Check sheet for the modelled part. Datum: model origin and axes. Units: mm. Face numbers are marked on the shaded views. A direction names the side the tool comes from. Give positions to 0.01 mm unless a question says otherwise; leave off trailing zeros. Loops run counter-clockwise (first coordinate to the right, second up) from the corner with the lowest first, then second, coordinate; pieces in that order, holes last. Notation, with made-up numbers: M -0.75,10 L 35.25,10 A25 cw 35.25,47 Z; hole C -23,6.5 d4. An arc over 180 degrees is marked long. Use one line per item in the form item = value.
Autodesk Inventor part; units mm, degrees
ref_plane "YZ Plane" through (0, 0, 0) normal (1, 0, 0) x (0, 1, 0)
ref_plane "XZ Plane" through (0, 0, 0) normal (0, 1, 0) x (-1, 0, 0)
ref_plane "XY Plane" through (0, 0, 0) normal (0, 0, 1) x (1, 0, 0)
sketch "Sketch1" plane through (0, 0, 0) normal (0, 1, 0) x (-1, 0, 0)
  line L0 (-8.75, 22.75) -> (8.75, 22.75)
  line L1 (8.75, 22.75) -> (8.75, -22.75)
  line L2 (8.75, -22.75) -> (-8.75, -22.75)
  line L3 (-8.75, -22.75) -> (-8.75, 22.75)
  line L4 (-8.75, 22.75) -> (8.75, -22.75) construction
  line L5 (8.75, 22.75) -> (-8.75, -22.75) construction
  line L6 (-1.6021, -2.775) -> (-3.2043, 0)
  line L7 (-3.2043, 0) -> (-1.6021, 2.775)
  line L8 (-1.6021, 2.775) -> (1.6021, 2.775)
  line L9 (1.6021, 2.775) -> (3.2043, 0)
  line L10 (3.2043, 0) -> (1.6021, -2.775)
  line L11 (1.6021, -2.775) -> (-1.6021, -2.775)
  line L12 (6.091, 0) -> (3.0455, 5.275)
  line L13 (3.0455, 5.275) -> (-3.0455, 5.275)
  line L14 (-3.0455, 5.275) -> (-6.091, 0)
  line L15 (-6.091, 0) -> (-3.0455, -5.275)
  line L16 (-3.0455, -5.275) -> (3.0455, -5.275)
  line L17 (3.0455, -5.275) -> (6.091, 0)
  line L18 (6.75, -20.75) -> (6.75, 20.75)
  line L19 (6.75, 20.75) -> (-6.75, 20.75)
  line L20 (-6.75, 20.75) -> (-6.75, -20.75)
  line L21 (-6.75, -20.75) -> (6.75, -20.75)
  circle A0 centre (0, 0) radius 1.6
  circle A1 centre (0, 0) radius 8.75
  circle A2 centre (0, 0) radius 6.75
  dimension "d0" = 17.5
  dimension "d1" = 45.5
  dimension "d2" = 5.55
  dimension "d8" = 2.5
  dimension "d9" = 2
  dimension "d11" = 3.2
  dimension "d14" = 17.5
  dimension "d15" = 2
extrude "Extrusion1" add sketch "Sketch1" along normal blind 5.95 contours A1 L20 | A1 L18 | A1 L18 A2 L20 | L20 A2 L18 A1 | A2 | L6 L7 L8 L9 L10 L11 | L17 L16 L15 L14 L13 L12 | A0
extrude "Extrusion5" add sketch "Sketch1" against normal blind 2 contours L6 L7 L8 L9 L10 L11 | L17 L16 L15 L14 L13 L12
extrude "Extrusion2" cut sketch "Sketch1" along normal blind 4 contours A2 | L6 L7 L8 L9 L10 L11 | A0
fillet "Fillet1" radius 1 6 edges at (6.091, 1, 0) (-3.0455, 1, 5.275) (3.0455, 1, -5.275) (-3.0455, 1, -5.275) (-6.091, 1, 0) (3.0455, 1, 5.275)
fillet "Fillet2" [suppressed]
equation "\"d14\" = d0"
properties part number "Solenoid Shield"
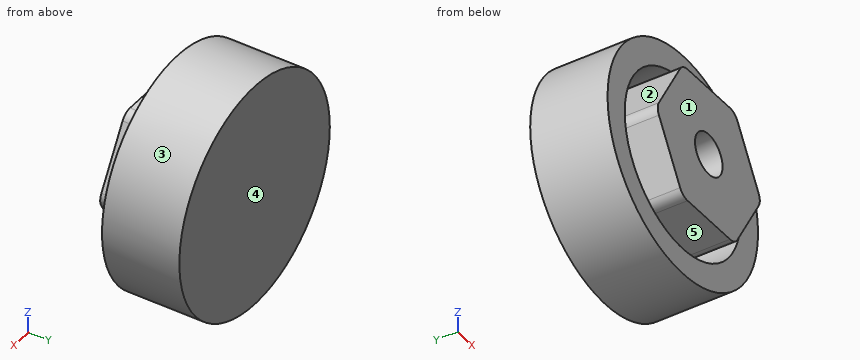
1) Section check B-B (z = 4.5). Record the cut outline in (x, y).
Evaluation:
outline = M -7.5,0 L -5.03,0 L -5.03,4 L -3.49,4 L -3.49,-2 L 3.49,-2 L 3.49,4 L 5.03,4 L 5.03,0 L 7.5,0 L 7.5,5.95 L -7.5,5.95 Z
2) Depth check by flat-ended pin: pin 1 Ø3.5 at (x, y) = (0.5, 2.5) entering from +Z; pin 2 Ø4 at (y, z) = (2.5, 5.5) entering from +X. Enter the tip coordinate at first touch or a pass-through.
Evaluation:
pin_1 = 8.75
pin_2 = 8.02
3) Scan lines: line 1 (Z direction, x = 5.5, y = 3); line 2 (X direction, y = 3.75, z = 4.75); line 3 (Z direction, x = 0, y = -0.6) (3 decimals). Record each from-to range of solid material in increasing order.
Evaluation:
line_1 = -6.81 to -3.91, -1.02 to 1.02, 3.91 to 6.81
line_2 = -7.35 to -4.8, -3.35 to 3.35, 4.8 to 7.35
line_3 = -5.275 to -1.6, 1.6 to 5.275
4) Section check D-D (x = -4.75). Record the cut outline in (y, z).
Evaluation:
outline = M -2,-2.32 L 4,-2.32 L 4,-4.8 L 0,-4.8 L 0,-7.35 L 5.95,-7.35 L 5.95,7.35 L 0,7.35 L 0,4.8 L 4,4.8 L 4,2.32 L -2,2.32 Z
5) Section check A-A (y = 2.25). Record the cut outline in (x, z) (3 decimals).
Evaluation:
outline = C 0,0 d17.5; M -5.802,-0.5 L -3.334,-4.775 A1 ccw -2.468,-5.275 L 2.468,-5.275 A1 ccw 3.334,-4.775 L 5.802,-0.5 A1 ccw 5.802,0.5 L 3.334,4.775 A1 ccw 2.468,5.275 L -2.468,5.275 A1 ccw -3.334,4.775 L -5.802,0.5 A1 ccw Z; hole C 0,0 d13.5; hole M -3.204,0 L -1.602,-2.775 L 1.602,-2.775 L 3.204,0 L 1.602,2.775 L -1.602,2.775 Z
6) Set-up check for the marked faces 4 and 5: record each of +Z, -Z, +X, -X, +Y, -Y from which the full face is reachable in a straight line by a thin tool's end or side.
Evaluation:
face_4 = +Z, -Z, +X, -X, +Y
face_5 = -Y
7) Section check C-C (x = 0). Record the cut outline in (y, z) (3 decimals).
Evaluation:
outline = M -2,-5.275 L 4,-5.275 L 4,-6.75 L 0,-6.75 L 0,-8.75 L 5.95,-8.75 L 5.95,8.75 L 0,8.75 L 0,6.75 L 4,6.75 L 4,5.275 L -2,5.275 L -2,1.6 L 0,1.6 L 0,2.775 L 4,2.775 L 4,-2.775 L 0,-2.775 L 0,-1.6 L -2,-1.6 Z
8) Release check for a two-part mould opening along Z. For the marked faces 1, 2 and 3 record: pulls with the +Z half, pulls with the -Z half, needs draft (parallel to the pull), parting line crosses it, or undercut.
Evaluation:
face_1 = needs draft
face_2 = undercut
face_3 = parting line crosses it
